CAD build for the part. Positions are in the model's coordinates, mm. A direction names the side the tool comes from. Coordinates: 2 decimals unless noted, no trailing zeros. Order: outer loops, then holes, each group sorted by start corner. A loop starts at its lowest first (then second) coordinate and runs counter-clockwise, first axis right, second up. Notation, with made-up numbers: M 52.25,0.25 L 83.25,0.25 A21 ccw 83.25,29.25 Z; hole C 65,-8 d11. An arc over 180 degrees is marked long. One line per item, written item: value.
from build123d import *

# Parameters (mm, degrees)
SKETCH1_RX          = 15
SKETCH1_RY          = 12.5
SKETCH1_W           = 6
SKETCH1_H           = 3.4
BOSS_EXTRUDE1_DEPTH = 5.85


with BuildPart() as part:
    # Sketch1 → Boss-Extrude1 (new body)
    with BuildSketch(Plane.XY):
        with BuildLine():
            Line((12.961794972, -22.772242018), (15.361794972, -22.772242018))
            Line((15.361794972, -22.772242018), (15.361794972, -21.547840006))
            Line((15.361794972, -21.547840006), (20, -21.547840006))
            Line((20, -21.547840006), (20, -28.31))
            Line((20, -28.31), (25, -28.31))
            Line((25, -28.31), (25, -31.69))
            Line((25, -31.69), (20, -31.69))
            ThreePointArc((20, -31.69), (0, -27.6), (-20, -31.69))
            Line((-20, -31.69), (-25, -31.69))
            Line((-25, -31.69), (-25, -28.31))
            Line((-25, -28.31), (-20, -28.31))
            Line((-20, -28.31), (-20, -21.547840006))
            Line((-20, -21.547840006), (-15.361794972, -21.547840006))
            Line((-15.361794972, -21.547840006), (-15.361794972, -22.772242018))
            Line((-15.361794972, -22.772242018), (-12.961794972, -22.772242018))
            Line((-12.961794972, -22.772242018), (-12.961794972, -21.547840006))
            Line((-12.961794972, -21.547840006), (-11.361794972, -21.547840006))
            Line((-11.361794972, -21.547840006), (-11.361794972, -18.452159994))
            Line((-11.361794972, -18.452159994), (-12.961794972, -18.452159994))
            Line((-12.961794972, -18.452159994), (-12.961794972, -17.227757982))
            Line((-12.961794972, -17.227757982), (-15.361794972, -17.227757982))
            Line((-15.361794972, -17.227757982), (-15.361794972, -18.452159994))
            Line((-15.361794972, -18.452159994), (-20, -18.452159994))
            Line((-20, -18.452159994), (-20, 0))
            Line((-20, 0), (-20, 18.452159994))
            Line((-20, 18.452159994), (-15.361794972, 18.452159994))
            Line((-15.361794972, 18.452159994), (-15.361794972, 17.227757982))
            Line((-15.361794972, 17.227757982), (-12.961794972, 17.227757982))
            Line((-12.961794972, 17.227757982), (-12.961794972, 18.452159994))
            Line((-12.961794972, 18.452159994), (-11.361794972, 18.452159994))
            Line((-11.361794972, 18.452159994), (-11.361794972, 21.547840006))
            Line((-11.361794972, 21.547840006), (-12.961794972, 21.547840006))
            Line((-12.961794972, 21.547840006), (-12.961794972, 22.772242018))
            Line((-12.961794972, 22.772242018), (-15.361794972, 22.772242018))
            Line((-15.361794972, 22.772242018), (-15.361794972, 21.547840006))
            Line((-15.361794972, 21.547840006), (-20, 21.547840006))
            Line((-20, 21.547840006), (-20, 28.31))
            Line((-20, 28.31), (-25, 28.31))
            Line((-25, 28.31), (-25, 31.69))
            Line((-25, 31.69), (-20, 31.69))
            ThreePointArc((-20, 31.69), (0, 27.6), (20, 31.69))
            Line((20, 31.69), (25, 31.69))
            Line((25, 31.69), (25, 28.31))
            Line((25, 28.31), (20, 28.31))
            Line((20, 28.31), (20, 21.547840006))
            Line((20, 21.547840006), (15.361794972, 21.547840006))
            Line((15.361794972, 21.547840006), (15.361794972, 22.772242018))
            Line((15.361794972, 22.772242018), (12.961794972, 22.772242018))
            Line((12.961794972, 22.772242018), (12.961794972, 21.547840006))
            Line((12.961794972, 21.547840006), (11.361794972, 21.547840006))
            Line((11.361794972, 21.547840006), (11.361794972, 18.452159994))
            Line((11.361794972, 18.452159994), (12.961794972, 18.452159994))
            Line((12.961794972, 18.452159994), (12.961794972, 17.227757982))
            Line((12.961794972, 17.227757982), (15.361794972, 17.227757982))
            Line((15.361794972, 17.227757982), (15.361794972, 18.452159994))
            Line((15.361794972, 18.452159994), (20, 18.452159994))
            Line((20, 18.452159994), (20, 0))
            Line((20, 0), (20, -18.452159994))
            Line((20, -18.452159994), (15.361794972, -18.452159994))
            Line((15.361794972, -18.452159994), (15.361794972, -17.227757982))
            Line((15.361794972, -17.227757982), (12.961794972, -17.227757982))
            Line((12.961794972, -17.227757982), (12.961794972, -18.452159994))
            Line((12.961794972, -18.452159994), (11.361794972, -18.452159994))
            Line((11.361794972, -18.452159994), (11.361794972, -21.547840006))
            Line((11.361794972, -21.547840006), (12.961794972, -21.547840006))
            Line((12.961794972, -21.547840006), (12.961794972, -22.772242018))
        make_face()
        with Locations(Location((0, 0), (0, 0, 90))):
            Ellipse(SKETCH1_RX, SKETCH1_RY, mode=Mode.SUBTRACT)
        with Locations((-4, 21.3)):
            Rectangle(SKETCH1_W, SKETCH1_H, mode=Mode.SUBTRACT)
        with Locations((-4, -21.3)):
            Rectangle(SKETCH1_W, SKETCH1_H, mode=Mode.SUBTRACT)
    extrude(amount=BOSS_EXTRUDE1_DEPTH)


solid = part.part
Q1. Pin check, flat tips, straight feed: pin 1 Ø0.6 at (y, z) = (22, 4) entering from -X; pin 2 Ø1.2 at (x, z) = (-14, 4) entering from +Y; pin 3 Ø1.3 at (x, z) = (12, 3) entering from +Y. Stop position of each tip, or through.
Recorded:
pin 1: stops at x = -20
pin 2: stops at y = 29.74
pin 3: stops at y = 29.2
Q2. Mould opens along Y. For faces 4 (the face through (-23, 31.69, 3)), 5 (the face through (-25, -30, 3)), 6 (the face through (-4, -19.6, 3)) say: released by +Y, released by -Y, zero draft, split by the parting line, or undercut.
Recorded:
face 4: released by +Y
face 5: zero draft
face 6: undercut
Q3. Slice it at A-A (y = 20.5). List the corners of the cut face in (x, z).
Recorded:
outline: M -11.36,0 L -7,0 L -7,5.85 L -11.36,5.85 Z; M -1,0 L 11.36,0 L 11.36,5.85 L -1,5.85 Z
Q4. Slice it at B-B (z = 4.15). Give the number of separate pieces and of enclosed holes in the cut face, plus the area to 3 significant figures.
Recorded:
separate pieces: 1
enclosed holes: 3
area: 1,620 mm^2
Q5. Which spindle directions (+Z, -Z, +X, -X, +Y, -Y) get a long thin tool onto all of the face, cutting with end or side? Do faces 1 (the face through (-4, 19.6, 3)), 2 (the face through (-12, -21.548, 3)), 3 (the face through (12, -21.548, 3)). Say none if no direction does.
Recorded:
face 1: +Z, -Z
face 2: +Z, -Z, -X
face 3: +Z, -Z, +X
Q6. Drill centre lines: line 1 along Y through (x, z) = (21, 1.65); line 2 along Y through (x, z) = (19.5, 3.3); line 3 along Y through (x, z) = (-14, 1.05). Where is each one in solid material? Low to high.
Recorded:
line 1: y = -31.69 to -28.31, 28.31 to 31.69
line 2: y = -31.48 to -21.55, -18.45 to 18.45, 21.55 to 31.48
line 3: y = -29.56 to -22.77, -17.23 to 17.23, 22.77 to 29.56
